The drawing under review shows one solid part. Ordinate dimensions are in mm from its lowest x, y, z. A direction names the side the tool comes from. Give positions to 0.01 mm unless a question says otherwise; leave off trailing zeros. Return JSON: item names as keys, results as strings. Group by question number.
1) Insertion check: P1, Ø16.5, axis at x = 68.26, y = 9.84, coming from the -Z side; P2, Ø4, axis at x = 87.5, z = 86, coming from the +Y side; P3, Ø5, axis at x = 49.5, z = 86.5, coming from the -Y side (1 decimal). Each pin has a flat end and moves straight along its axis. Give the tip position at first contact, or say it passes through.
2) The part is to be moulded in two halves that separate along X. For the marked faces 3, 4 and 5, say which applies: released by +X, released by -X, zero draft, split by the parting line, or undercut.
3) To check wall thickness, follow line 1 along X through (y, z) = (67, 16) (1 decimal); line 2 along Y through (x, z) = (122.5, 83) (1 decimal); line 3 along Z through (x, y) = (13.5, 78.5). State the ranges of each line that lie inside material, in increasing order.
4) Add section A-A (z = 90.5). State how many separate pieces and enclosed holes the cut face has, then the cut area to 3 significant figures.
5) For the marked faces 1 and 2, list the 3-axis set-ups (+Z, -Z, +X, -X, +Y, -Y) from which the entire face can be reached by the end or side of a thin tool; tool diameter is ignored.
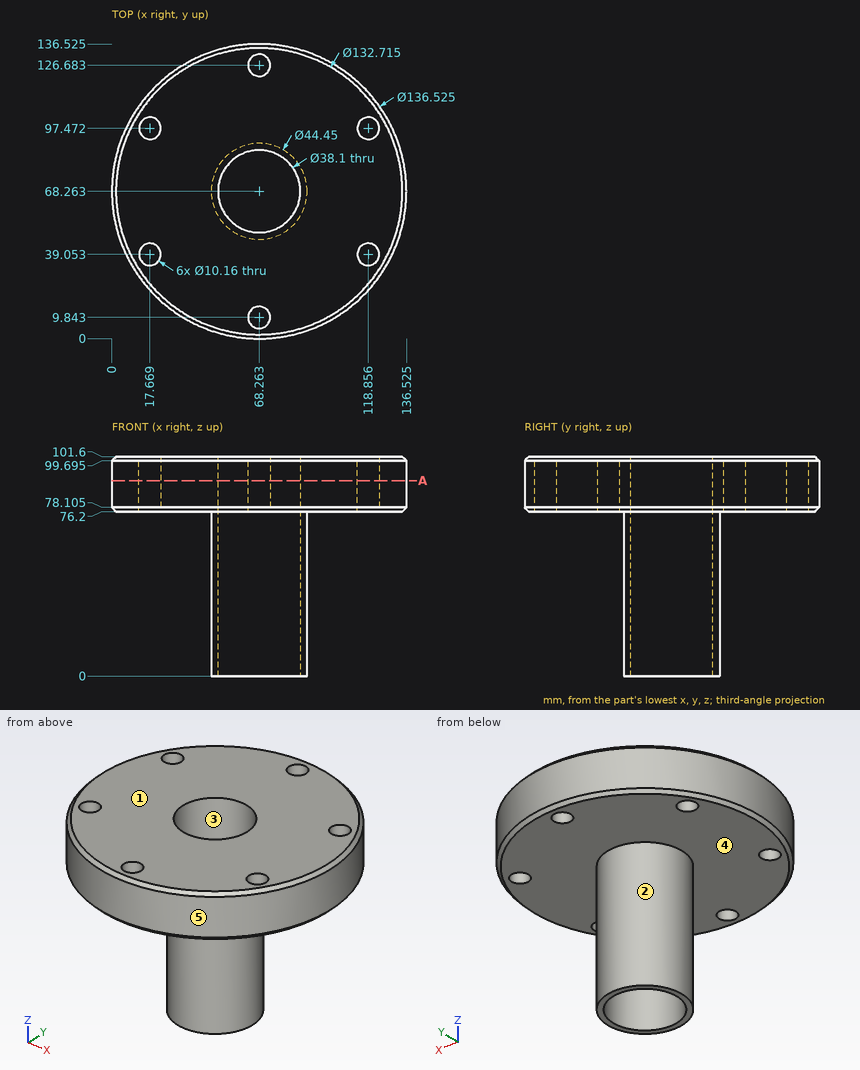
Evaluation:
{
 "1": {"P1": "z = 76.2", "P2": "y = 134.31", "P3": "y = 2"},
 "2": {"face 3": "undercut", "face 4": "zero draft", "face 5": "split by the parting line"},
 "3": {"line 1": "46.1 to 49.3, 87.3 to 90.5", "line 2": "26.8 to 35.5, 42.6 to 93.9, 101 to 109.7", "line 3": "76.2 to 101.6"},
 "4": {"separate pieces": "1", "enclosed holes": "7", "area": "13,000 mm^2"},
 "5": {"face 1": "+Z, +X, -X, +Y, -Y", "face 2": "-Z"}
}
